from build123d import *

# Parameters (mm, degrees)
SKETCH2_W           = 8
SKETCH2_H           = 15
SKETCH2_R           = 2
SKETCH2_W_2         = 42
SKETCH2_H_2         = 8
BOSS_EXTRUDE1_DEPTH = 3
SKETCH2_3_W         = 17
SKETCH2_3_H         = 15
BOSS_EXTRUDE2_DEPTH = 3
BOSS_EXTRUDE3_DEPTH = 5
SKETCH4_W           = 17
SKETCH4_H           = 1.9
BOSS_EXTRUDE4_DEPTH = 3
SKETCH5_R           = 1.5
CUT_EXTRUDE1_DEPTH  = 30.567718884
FILLET1_R           = 1
FILLET2_R           = 2


with BuildPart() as part:
    # Sketch2 → Boss-Extrude1 (new body)
    # profile 1 of 2: a face of its own
    with BuildSketch(Plane(origin=(0, 0, 0), x_dir=(1, 0, 0), z_dir=(0, 1, 0))):
        with Locations((0, 11.5)):
            Rectangle(SKETCH2_W, SKETCH2_H)
        with Locations(Location((0, 15, 0), (0, 0, 270))):
            Circle(SKETCH2_R, mode=Mode.SUBTRACT)
    # profile 2 of 2: a face of its own
    with BuildSketch(Plane(origin=(0, 0, 0), x_dir=(1, 0, 0), z_dir=(0, 1, 0))):
        Rectangle(SKETCH2_W_2, SKETCH2_H_2)
        with Locations(Location((17, 0, 0), (0, 0, 270))):
            Circle(SKETCH2_R, mode=Mode.SUBTRACT)
        with Locations(Location((-17, 0, 0), (0, 0, 270))):
            Circle(SKETCH2_R, mode=Mode.SUBTRACT)
        with Locations(Location((0, 0, 0), (0, 0, 270))):
            Circle(SKETCH2_R, mode=Mode.SUBTRACT)
    extrude(amount=BOSS_EXTRUDE1_DEPTH)

    # Sketch2_3 → Boss-Extrude2 (add)
    with BuildSketch(Plane(origin=(0, 0, 0), x_dir=(1, 0, 0), z_dir=(0, 1, 0))):
        with Locations((0, -11.5)):
            Rectangle(SKETCH2_3_W, SKETCH2_3_H)
    extrude(amount=BOSS_EXTRUDE2_DEPTH)

    # Sketch3 → Boss-Extrude3 (add)
    with BuildSketch(Plane.XY.offset(19)):
        with BuildLine():
            Line((-8.5, 11.5), (-14, 11.5))
            Line((-14, 11.5), (-14, 8.5))
            Line((-14, 8.5), (-8.5, 8.5))
            Line((-8.5, 8.5), (-8.5, 3))
            Line((-8.5, 3), (8.5, 3))
            Line((8.5, 3), (8.5, 8.5))
            Line((8.5, 8.5), (14, 8.5))
            Line((14, 8.5), (14, 11.5))
            Line((14, 11.5), (8.5, 11.5))
            Line((8.5, 11.5), (6.6, 11.5))
            ThreePointArc((6.6, 11.5), (0, 4.9), (-6.6, 11.5))
            Line((-6.6, 11.5), (-8.5, 11.5))
        make_face()
    extrude(amount=-BOSS_EXTRUDE3_DEPTH)

    # Sketch4 → Boss-Extrude4 (add)
    with BuildSketch(Plane(origin=(0, 0, 14), x_dir=(-1, 0, 0), z_dir=(0, 0, -1))):
        with Locations((0, 3.95)):
            Rectangle(SKETCH4_W, SKETCH4_H)
    extrude(amount=BOSS_EXTRUDE4_DEPTH)

    # Sketch5 → Cut-Extrude1 (cut, through all)
    with BuildSketch(Plane.XZ.offset(-8.5)):
        with Locations(Location((11.5, 16.5, 0), (0, 0, 270))):
            Circle(SKETCH5_R)
        with Locations(Location((-11.5, 16.5, 0), (0, 0, 90))):
            Circle(SKETCH5_R)
    extrude(amount=-CUT_EXTRUDE1_DEPTH, mode=Mode.SUBTRACT)

    # Fillet1
    fillet1_edges = [part.edges().sort_by_distance(p)[0] for p in [
        (-6.6, 11.5, 16.5),
        (6.6, 11.5, 16.5),
    ]]
    fillet(fillet1_edges, radius=FILLET1_R)

    # Fillet2
    fillet2_edges = [part.edges().sort_by_distance(p)[0] for p in [
        (4, 1.5, -4),
        (21, 1.5, -4),
        (21, 1.5, 4),
        (-21, 1.5, 4),
        (-21, 1.5, -4),
        (-4, 1.5, -4),
        (-4, 1.5, -19),
        (4, 1.5, -19),
        (8.5, 1.5, 4),
        (-8.5, 1.5, 4),
    ]]
    fillet(fillet2_edges, radius=FILLET2_R)


solid = part.part
For this review, take the finished solid that the model builds, in its own axes (mm). A direction names the side the tool comes from. Give positions to 0.01 mm unless a question says otherwise; leave off trailing zeros. Loops run counter-clockwise (first coordinate to the right, second up) from the corner with the lowest first, then second, coordinate; pieces in that order, holes last.
Item 1: Take a section at A-A, the plane x = -11.5. State the section outline as (y, z) points.
Item 2: Take a section at C-C, the plane y = 2. State the section outline as (x, z) points.
Item 3: Take a section at B-B, the plane z = 0. State the section outline as (x, y) points, and give its area (3 significant figures).
Item 4: Draft analysis for pull direction Z (two halves, no side actions). For faces 4 (the cylindrical face through (-20.4, 1.52, 3.43)), 5 (the flat face through (10, 8.5, 18)), 6 (the cylindrical face through (-2, 1, 0)), 7 (the flat face through (0, 1, -19)), state which applies: +Z half, -Z half, draft (parallel to the pull), parting line (faces both ways), or undercut.
Item 5: Tool access review of faces 1 (the flat face through (-15, 1, 4)), 2 (the cylindrical face through (6.87, 11.25, 16.46)), 3 (the flat face through (15, 1, 4)): name each direction out of +Z, -Z, +X, -X, +Y, -Y from which nothing blocks a thin tool from reaching the whole face with its end or side.
Item 6: Take a section at D-D, the plane x = 17. State the section outline as (y, z) points, and give its area (3 significant figures).
Item 7: Insertion check: pin 1 (3.5 mm diameter, centred on x = 15.5, y = 1.5, fed in from -Z); pin 2 (2.5 mm diameter, centred on x = -10.5, z = 17.5, fed in from -Y); pin 3 (2.5 mm diameter, centred on y = 10, z = 17, fed in from +X). Each pin has a flat end and moves straight along its axis. Give the tip position at first contact, or say it passes through.
Item 8: For line 1 along X through (y, z) = (2.2, 0); line 2 along Z through (x, y) = (-11.5, 9.9); line 3 along X through (y, z) = (10.7, 16.5), list the stretches that pass through material, from the lowest coordinate up.
Calculated:
1. outline: (0, -4) - (3, -4) - (3, 4) - (0, 4) - close; (8.5, 14) - (11.5, 14) - (11.5, 15) - (8.5, 15) - close; (8.5, 18) - (11.5, 18) - (11.5, 19) - (8.5, 19) - close
2. outline: (-21, -2) arc R2 ccw to (-19, -4) - (-6, -4) arc R2 cw to (-4, -6) - (-4, -17) arc R2 ccw to (-2, -19) - (2, -19) arc R2 ccw to (4, -17) - (4, -6) arc R2 cw to (6, -4) - (19, -4) arc R2 ccw to (21, -2) - (21, 2) arc R2 ccw to (19, 4) - (10.5, 4) arc R2 cw to (8.5, 6) - (8.5, 19) - (-8.5, 19) - (-8.5, 6) arc R2 cw to (-10.5, 4) - (-19, 4) arc R2 ccw to (-21, 2) - close; hole circle Ø4 at (-17, 0); hole circle Ø4 at (0, -15); hole circle Ø4 at (0, 0); hole circle Ø4 at (17, 0)
3. outline: (-21, 0) - (-19, 0) - (-19, 3) - (-21, 3) - close; (-15, 0) - (-2, 0) - (-2, 3) - (-15, 3) - close; (2, 0) - (15, 0) - (15, 3) - (2, 3) - close; (19, 0) - (21, 0) - (21, 3) - (19, 3) - close
3. area: 90.0 mm2
4. face 4: +Z half
4. face 5: draft
4. face 6: undercut
4. face 7: -Z half
5. face 1: +Z, -X, +Y, -Y
5. face 2: +Z, -Z, +Y
5. face 3: +Z, +X, +Y, -Y
6. outline: (0, -4) - (3, -4) - (3, -2) - (0, -2) - close; (0, 2) - (3, 2) - (3, 4) - (0, 4) - close
6. area: 12.0 mm2
7. pin 1: stops at z = -4
7. pin 2: stops at y = 8.5
7. pin 3: stops at x = 14
8. line 1: x = -21 to -19, -15 to -2, 2 to 15, 19 to 21
8. line 2: z = 14 to 15, 18 to 19
8. line 3: x = -14 to -13, -10 to -6.55, 6.55 to 10, 13 to 14
